The listing builds one solid part. Answer for the finished solid, in the listing's coordinates (mm). A direction names the side the tool comes from. Round coordinates to 2 decimals unless told otherwise and drop trailing zeros. Write each loop counter-clockwise with the first axis right and the second up, starting at its lowest first coordinate (ties: lowest second). Pieces come first, ordered by that corner, then holes. Notation, with made-up numbers: (52, -26.75) - (103, -26.75) arc R26 ccw to (103, -5.75) - close; hole circle Ø5 at (4.25, 37.5). An arc over 180 degrees is marked (long way). Return JSON: item names as keys, results as strings. Group by question number.
(1) Section B-B, the plane y = 0 is taken. Write down the section's boundary in (x, z), then the cut area to 3 significant figures.
(2) Which of the six approach directions +Z, -Z, +X, -X, +Y, -Y give full straight-line access (tool end or side, diameter ignored) to faces 5 (the flat face through (-0.013, 3.356, 0.021)), 6 (the flat face through (-0.9, -4, 0))?
(3) Find the intervals of material crossed by line 1 along Z through (x, y) = (0.1, 0.25); line 2 along Z through (x, y) = (0.4, 3); line 3 along Y through (x, z) = (0.4, -1), in increasing order. Write a range as [from, to].
(4) Determine the mould class of faces 1 (the cylindrical face through (0.013, 1.802, -5.723)), 2 (the flat face through (0.9, -4, 0)), 3 (the flat face through (-0.013, -3.356, -0.021)), 4 (the cylindrical face through (0, 0.1, 4.1)) for opening direction Y: +Y half, -Y half, draft (parallel to the pull), parting line (faces both ways), or undercut.
(5) Section D-D, the plane x = 0.45 is taken. Write down the section's boundary in (y, z), then the cut area to 3 significant figures.
(6) Section C-C, the plane x = -0.2 is taken. Write down the section's boundary in (y, z), then the cut area to 3 significant figures.
(7) Section A-A, the plane z = 0 is taken. Write down the section's boundary in (x, y), then the cut area to 3 significant figures.
```python
from build123d import *

# Parameters (mm, degrees)
SKETCH1_R                     = 6
SKETCH1_R_2                   = 4.1
BOSS_EXTRUDE1_DEPTH           = 0.9
BOSS_EXTRUDE2_START           = -0.9
BOSS_EXTRUDE2_DEPTH           = 1.8
BOSS_EXTRUDE2_DRAFT           = 10
BOSS_EXTRUDE2_PROFILE_2_DEPTH = 1.8
BOSS_EXTRUDE2_PROFILE_2_DRAFT = 10


with BuildPart() as part:
    # Sketch1 → Boss-Extrude1 (new, symmetric)
    with BuildSketch(Plane.YZ):
        with Locations(Location((0, 0, 0), (0, 0, 270))):
            Circle(SKETCH1_R)
        with Locations(Location((0, 0, 0), (0, 0, 270))):
            Circle(SKETCH1_R_2, mode=Mode.SUBTRACT)
    extrude(amount=BOSS_EXTRUDE1_DEPTH, both=True)


with BuildPart() as boss_extrude2_tool:
    # Sketch2 → Boss-Extrude2 (with draft: the straight prism first)
    with BuildSketch(Plane.YZ.offset(BOSS_EXTRUDE2_START)):
        with BuildLine():
            Line((5.809475019, 1.5), (3.2, 1.5))
            Line((3.2, 1.5), (3.2, -1.5))
            Line((3.2, -1.5), (5.809475019, -1.5))
            ThreePointArc((5.809475019, -1.5), (6, 0), (5.809475019, 1.5))
        make_face()
    extrude(amount=BOSS_EXTRUDE2_DEPTH)
    # Boss-Extrude2: the draft: its side faces are tilted about the plane it starts from
    boss_extrude2_sides = [boss_extrude2_tool.faces().sort_by_distance(p)[0] for p in [
        (0, 4.50473751, 1.5),
        (0, 3.2, 0),
        (0, 4.50473751, -1.5),
        (0, 6, 0),
    ]]
    draft(boss_extrude2_sides, Plane.YZ.offset(BOSS_EXTRUDE2_START), BOSS_EXTRUDE2_DRAFT)


with BuildPart() as part_1:
    add(part.part)

    # Boss-Extrude2: add boss_extrude2_tool
    add(boss_extrude2_tool.part)


with BuildPart() as boss_extrude2_profile_2_tool:
    # Sketch2 → Boss-Extrude2 profile 2 (with draft: the straight prism first)
    with BuildSketch(Plane.YZ.offset(BOSS_EXTRUDE2_START)):
        with BuildLine():
            ThreePointArc((-5.809475019, 1.5), (-6, 0), (-5.809475019, -1.5))
            Line((-5.809475019, -1.5), (-3.2, -1.5))
            Line((-3.2, -1.5), (-3.2, 1.5))
            Line((-3.2, 1.5), (-5.809475019, 1.5))
        make_face()
    extrude(amount=BOSS_EXTRUDE2_PROFILE_2_DEPTH)
    # Boss-Extrude2 profile 2: the draft: its side faces are tilted about the plane it starts from
    boss_extrude2_profile_2_sides = [boss_extrude2_profile_2_tool.faces().sort_by_distance(p)[0] for p in [
        (0, -6, 0),
        (0, -4.50473751, -1.5),
        (0, -3.2, 0),
        (0, -4.50473751, 1.5),
    ]]
    draft(boss_extrude2_profile_2_sides, Plane.YZ.offset(BOSS_EXTRUDE2_START), BOSS_EXTRUDE2_PROFILE_2_DRAFT)


with BuildPart() as part_2:
    add(part_1.part)

    # Boss-Extrude2 profile 2: add boss_extrude2_profile_2_tool
    add(boss_extrude2_profile_2_tool.part)


solid = part_2.part
```
Working result:
{
 "1": {"outline": "(-0.9, -6) - (0.9, -6) - (0.9, -4.1) - (-0.9, -4.1) - close; (-0.9, 4.1) - (0.9, 4.1) - (0.9, 6) - (-0.9, 6) - close", "area": "6.84 mm^2"},
 "2": {"face 5": "+X", "face 6": "+Z, -Z, -X, +Y, -Y"},
 "3": {"line 1": "z = [-5.99, -4.09], [4.09, 5.99]", "line 2": "z = [-5.2, -2.79], [2.79, 5.2]", "line 3": "y = [-5.92, -3.43], [3.43, 5.92]"},
 "4": {"face 1": "parting line", "face 2": "draft", "face 3": "undercut", "face 4": "undercut"},
 "5": {"outline": "circle Ø12 at (0, 0); hole (-3.9, -1.26) arc R4.1 ccw to (3.9, -1.26) - (3.44, -1.26) - (3.44, 1.26) - (3.9, 1.26) arc R4.1 ccw to (-3.9, 1.26) - (-3.44, 1.26) - (-3.44, -1.26) - close", "area": "63.3 mm^2"},
 "6": {"outline": "circle Ø12 at (0, 0); hole (-3.86, -1.38) arc R4.1 ccw to (3.86, -1.38) - (3.32, -1.38) - (3.32, 1.38) - (3.86, 1.38) arc R4.1 ccw to (-3.86, 1.38) - (-3.32, 1.38) - (-3.32, -1.38) - close", "area": "64.1 mm^2"},
 "7": {"outline": "(-0.9, -6) - (0.9, -6) - (0.9, -3.52) - (-0.9, -3.2) - close; (-0.9, 3.2) - (0.9, 3.52) - (0.9, 6) - (-0.9, 6) - close", "area": "9.51 mm^2"}
}
